Check sheet for the modelled part. Datum: model origin and axes. Units: mm. A direction names the side the tool comes from. Round coordinates to 2 decimals unless told otherwise and drop trailing zeros. Order: outer loops, then holes, each group sorted by start corner. A loop starts at its lowest first (then second) coordinate and runs counter-clockwise, first axis right, second up. Notation, with made-up numbers: M 49,-18.75 L 106,-18.75 A22 cw 106,2.25 Z; hole C 30.5,-4 d10. An arc over 180 degrees is marked long. One line per item, written item: value. Start each with the question number.
(1) Cross-section at C-C, the plane x = 15. Enter the section's corners in (y, z) (3 decimals), and give its area (3 significant figures).
(2) Thickness scan on L1, parallel to Y at x = -17, z = -6.75 (3 decimals); L2, parallel to X at y = 2.5, z = 31; L3, parallel to X at y = -15, z = -4. Record the ranges inside material, lowest first.
(3) Release check for a two-part mould opening along X. For faces 4 (the face through (-25.4, 1, 11)), 5 (the face through (0, 5, 53.975)), 6 (the face through (-17.65, -18.93, -4.7)), 7 (the face through (25.4, 1, 11)) record: released by +X, released by -X, zero draft, split by the parting line, or undercut.
(4) Access from +Z, -Z, +X, -X, +Y, -Y to the whole of each face (thin tool, end or side, straight path). Record for faces 1 (the face through (-20, 5, 24)), 2 (the face through (0, -53.975, -5)), 3 (the face through (0, 0, 27)).
(5) Cross-section at A-A, the plane y = -16. Enter the section's corners in (x, z) (3 decimals).
(6) Depth check by flat-ended pin: pin 1 Ø5 at (x, z) = (-7, 43.5) entering from -Y; pin 2 Ø2 at (x, y) = (18, -32) entering from +Z. Enter the tip coordinate at first touch or a pass-through.
(7) Cross-section at B-B, the plane z = 35. Enter the section's corners in (x, y) (3 decimals), and give its area (3 significant figures).
(8) Cross-section at D-D, the plane z = -1. Enter the section's corners in (x, y) (3 decimals).
from build123d import *

# Parameters (mm, degrees)
F0_W     = 9.525
F0_H     = 53.975
F3_DEPTH = 25.4
F4_DEPTH = 9.526
F2_R     = 3
F5_DEPTH = 9.526


with BuildPart() as f3:
    # F0 (on Right) → F3 (new body, symmetric)
    with BuildSketch(Plane.YZ):
        Polygon((9.525, 0), (0, 0), (-53.975, 0), (-53.975, -9.525), (9.525, -9.525), align=None)
        with Locations((4.7625, 26.9875)):
            Rectangle(F0_W, F0_H)
    extrude(amount=F3_DEPTH, both=True)

    # F1 (on Front) → F4 (cut, through all)
    with BuildSketch(Plane.XZ):
        with BuildLine():
            ThreePointArc((-14, 6), (-14.87868, 8.12132), (-17, 9))
            Line((-17, 9), (-17, 3))
            ThreePointArc((-17, 3), (-14.87868, 3.87868), (-14, 6))
        make_face()
        with BuildLine():
            Line((-17, 3), (-17, 9))
            ThreePointArc((-17, 9), (-19.12132, 8.12132), (-20, 6))
            ThreePointArc((-20, 6), (-19.12132, 3.87868), (-17, 3))
        make_face()
        with BuildLine():
            Line((-17, 9), (-17, 39))
            ThreePointArc((-17, 39), (-19.12132, 39.87868), (-20, 42))
            Line((-20, 42), (-20, 6))
            ThreePointArc((-20, 6), (-19.12132, 8.12132), (-17, 9))
        make_face()
        with BuildLine():
            ThreePointArc((-14, 42), (-14.87868, 39.87868), (-17, 39))
            Line((-17, 39), (-17, 9))
            ThreePointArc((-17, 9), (-14.87868, 8.12132), (-14, 6))
            Line((-14, 6), (-14, 42))
        make_face()
        with BuildLine():
            ThreePointArc((-14, 42), (-14.87868, 44.12132), (-17, 45))
            Line((-17, 45), (-17, 39))
            ThreePointArc((-17, 39), (-14.87868, 39.87868), (-14, 42))
        make_face()
        with BuildLine():
            Line((-17, 39), (-17, 45))
            ThreePointArc((-17, 45), (-19.12132, 44.12132), (-20, 42))
            ThreePointArc((-20, 42), (-19.12132, 39.87868), (-17, 39))
        make_face()
        with BuildLine():
            ThreePointArc((20, 42), (19.12132, 44.12132), (17, 45))
            Line((17, 45), (17, 39))
            ThreePointArc((17, 39), (19.12132, 39.87868), (20, 42))
        make_face()
        with BuildLine():
            Line((17, 39), (17, 45))
            ThreePointArc((17, 45), (14.87868, 44.12132), (14, 42))
            ThreePointArc((14, 42), (14.87868, 39.87868), (17, 39))
        make_face()
        with BuildLine():
            Line((17, 9), (17, 39))
            ThreePointArc((17, 39), (14.87868, 39.87868), (14, 42))
            Line((14, 42), (14, 6))
            ThreePointArc((14, 6), (14.87868, 8.12132), (17, 9))
        make_face()
        with BuildLine():
            ThreePointArc((20, 42), (19.12132, 39.87868), (17, 39))
            Line((17, 39), (17, 9))
            ThreePointArc((17, 9), (19.12132, 8.12132), (20, 6))
            Line((20, 6), (20, 42))
        make_face()
        with BuildLine():
            ThreePointArc((20, 6), (19.12132, 8.12132), (17, 9))
            Line((17, 9), (17, 3))
            ThreePointArc((17, 3), (19.12132, 3.87868), (20, 6))
        make_face()
        with BuildLine():
            Line((17, 3), (17, 9))
            ThreePointArc((17, 9), (14.87868, 8.12132), (14, 6))
            ThreePointArc((14, 6), (14.87868, 3.87868), (17, 3))
        make_face()
    extrude(amount=-F4_DEPTH, mode=Mode.SUBTRACT)

    # F2 (on Top) → F5 (cut, through all)
    with BuildSketch(Plane.XY):
        with Locations((-17, -16)):
            Circle(F2_R)
        with Locations((17, -16)):
            Circle(F2_R)
    extrude(amount=-F5_DEPTH, mode=Mode.SUBTRACT)


solid = f3.part
Values found:
1. outline: M -53.975,-9.525 L -18.236,-9.525 L -18.236,0 L -53.975,0 Z; M -13.764,-9.525 L 9.525,-9.525 L 9.525,3.764 L 0,3.764 L 0,0 L -13.764,0 Z; M 0,44.236 L 9.525,44.236 L 9.525,53.975 L 0,53.975 Z
1. area: 691 mm^2
2. L1: -53.975 to -19, -13 to 9.525
2. L2: -25.4 to -20, -14 to 14, 20 to 25.4
2. L3: -25.4 to -19.83, -14.17 to 14.17, 19.83 to 25.4
3. face 4: released by -X
3. face 5: zero draft
3. face 6: undercut
3. face 7: released by +X
4. face 1: +Y, -Y
4. face 2: +Z, -Z, +X, -X, -Y
4. face 3: +Z, +X, -X, -Y
5. outline: M -25.4,-9.525 L -20,-9.525 L -20,0 L -25.4,0 Z; M -14,-9.525 L 14,-9.525 L 14,0 L -14,0 Z; M 20,-9.525 L 25.4,-9.525 L 25.4,0 L 20,0 Z
6. pin 1: y = 0
6. pin 2: z = 0
7. outline: M -25.4,0 L -20,0 L -20,9.525 L -25.4,9.525 Z; M -14,0 L 14,0 L 14,9.525 L -14,9.525 Z; M 20,0 L 25.4,0 L 25.4,9.525 L 20,9.525 Z
7. area: 370 mm^2
8. outline: M -25.4,-53.975 L 25.4,-53.975 L 25.4,9.525 L -25.4,9.525 Z; hole C -17,-16 d6; hole C 17,-16 d6
